```python
from build123d import *

# Parameters (mm, degrees)
BOSS_EXTRUDE1_DEPTH = 3
SKETCH3_R           = 1.5
BOSS_EXTRUDE2_DEPTH = 3
SKETCH4_R           = 1.5
CUT_EXTRUDE1_DEPTH  = 3


with BuildPart() as part:
    # Sketch2 → Boss-Extrude1 (new body)
    with BuildSketch(Plane.XY):
        with BuildLine():
            Line((-25.866686, 11.924208702), (-25.866686, 14.924208702))
            Line((-25.866686, 14.924208702), (-24.866686, 14.924208702))
            ThreePointArc((-24.866686, 14.924208702), (-29.366686, 13.424208702), (-24.866686, 11.924208702))
            Line((-24.866686, 11.924208702), (-25.866686, 11.924208702))
        make_face()
        with BuildLine():
            Line((-24.866686, 14.924208702), (-25.866686, 14.924208702))
            Line((-25.866686, 14.924208702), (-25.866686, 11.924208702))
            Line((-25.866686, 11.924208702), (-24.866686, 11.924208702))
            ThreePointArc((-24.866686, 11.924208702), (-24.494977755, 12.633639287), (-24.366686, 13.424208702))
            ThreePointArc((-24.366686, 13.424208702), (-24.494977755, 14.214778117), (-24.866686, 14.924208702))
        make_face()
        with BuildLine():
            Line((-18.866686, 14.924208702), (-24.866686, 14.924208702))
            ThreePointArc((-24.866686, 14.924208702), (-24.494977755, 14.214778117), (-24.366686, 13.424208702))
            ThreePointArc((-24.366686, 13.424208702), (-24.494977755, 12.633639287), (-24.866686, 11.924208702))
            Line((-24.866686, 11.924208702), (-18.866686, 11.924208702))
            ThreePointArc((-18.866686, 11.924208702), (-19.366686, 13.424208702), (-18.866686, 14.924208702))
        make_face()
        with BuildLine():
            ThreePointArc((-14.366686, 13.424208702), (-16.076116585, 15.795916947), (-18.866686, 14.924208702))
            Line((-18.866686, 14.924208702), (-17.866686, 14.924208702))
            Line((-17.866686, 14.924208702), (-17.866686, 11.924208702))
            Line((-17.866686, 11.924208702), (-18.866686, 11.924208702))
            ThreePointArc((-18.866686, 11.924208702), (-16.076116585, 11.052500457), (-14.366686, 13.424208702))
        make_face()
        with BuildLine():
            Line((-17.866686, 14.924208702), (-18.866686, 14.924208702))
            ThreePointArc((-18.866686, 14.924208702), (-19.366686, 13.424208702), (-18.866686, 11.924208702))
            Line((-18.866686, 11.924208702), (-17.866686, 11.924208702))
            Line((-17.866686, 11.924208702), (-17.866686, 14.924208702))
        make_face()
    extrude(amount=BOSS_EXTRUDE1_DEPTH)

    # Sketch3 → Boss-Extrude2 (add)
    with BuildSketch(Plane.XY.offset(3)):
        with Locations((-26.866686, 13.424208702)):
            Circle(SKETCH3_R)
    extrude(amount=BOSS_EXTRUDE2_DEPTH)

    # Sketch4 → Cut-Extrude1 (cut)
    with BuildSketch(Plane(origin=(0, 0, 0), x_dir=(-1, 0, 0), z_dir=(0, 0, -1))):
        with Locations((16.866686, 13.424208702)):
            Circle(SKETCH4_R)
    extrude(amount=-CUT_EXTRUDE1_DEPTH, mode=Mode.SUBTRACT)


solid = part.part
```
Geometry: final body of the model. Coordinates: model frame, mm. A direction names the side the tool comes from. Coordinates: 2 decimals unless noted, no trailing zeros. Order: outer loops, then holes, each group sorted by start corner. A loop starts at its lowest first (then second) coordinate and runs counter-clockwise, first axis right, second up. Notation, with made-up numbers: (82.5, 57.5) -> (128.5, 57.5) arc R18 ccw to (128.5, 63.5) -> close; hole circle Ø8 at (-32, 49). An arc over 180 degrees is marked (long way). Write each question's results on one line, items separated by ' | '. Start each with the question number.
1) Material intervals for line 1 along Z through (x, y) = (-24.25, 12.15); line 2 along X through (y, z) = (11.45, 1.1); line 3 along X through (y, z) = (15.6, 0.5), sorted ascending.
2) Cut plane A-A, the plane y = 13. Output: boundary loops of the cut face in (x, z).
3) Mould query, pull axis X, two halves, no side actions, for faces 3 (the flat face through (-22, 11.924, 1)), 4 (the cylindrical face through (-27.19, 11.96, 4.48)), 5 (the flat face through (-22, 13, 3)). Classes: released by +X, released by -X, zero draft, split by the parting line, or undercut.
4) Set-up query: faces 1 (the flat face through (-22, 14.924, 1)), 2 (the flat face through (-27, 13, 6)). Return all of +Z, -Z, +X, -X, +Y, -Y with unobstructed straight access to the full face (end or side cutting, diameter ignored); none if empty.
5) Cut plane B-B, the plane z = 1.35. Output: boundary loops of the cut face in (x, y).
6) First-contact query: pin 1 (0.9 mm diameter, centred on x = -21.5, z = 1, fed in from +Y); pin 2 (2 mm diameter, centred on x = -25.5, z = 5, fed in from -Y); pin 3 (0.9 mm diameter, centred on x = -20.5, z = 2, fed in from -Y); pin 4 (1 mm diameter, centred on x = -17, z = 3, fed in from -Y). Flat tips, straight axial feed; report the tip coordinate or a pass-through.
7) Cut plane D-D, the plane x = -20.25. Output: boundary loops of the cut face in (y, z), and give its area (3 significant figures).
8) Cut plane C-C, the plane x = -17.5. Output: boundary loops of the cut face in (y, z), and give its area (3 significant figures).
Checks:
1) line 1: 0 to 3 | line 2: -28.4 to -25.33, -18.4 to -15.33 | line 3: -28.1 to -25.64, -18.1 to -15.64
2) outline: (-29.33, 0) -> (-18.31, 0) -> (-18.31, 3) -> (-25.43, 3) -> (-25.43, 6) -> (-28.31, 6) -> (-28.31, 3) -> (-29.33, 3) -> close; (-15.43, 0) -> (-14.4, 0) -> (-14.4, 3) -> (-15.43, 3) -> close
3) face 3: undercut | face 4: split by the parting line | face 5: zero draft
4) face 1: +Z, -Z, +Y | face 2: +Z, +X, -X, +Y, -Y
5) outline: (-24.87, 11.92) -> (-18.87, 11.92) arc R2.5 ccw (long way) to (-18.87, 14.92) -> (-24.87, 14.92) arc R2.5 ccw (long way) to start; hole circle Ø3 at (-16.87, 13.42)
6) pin 1: y = 14.92 | pin 2: y = 11.97 | pin 3: y = 11.92 | pin 4: y = 10.92
7) outline: (11.92, 0) -> (14.92, 0) -> (14.92, 3) -> (11.92, 3) -> close | area: 9.00 mm^2
8) outline: (11.01, 0) -> (12.06, 0) -> (12.06, 3) -> (11.01, 3) -> close; (14.78, 0) -> (15.84, 0) -> (15.84, 3) -> (14.78, 3) -> close | area: 6.35 mm^2
